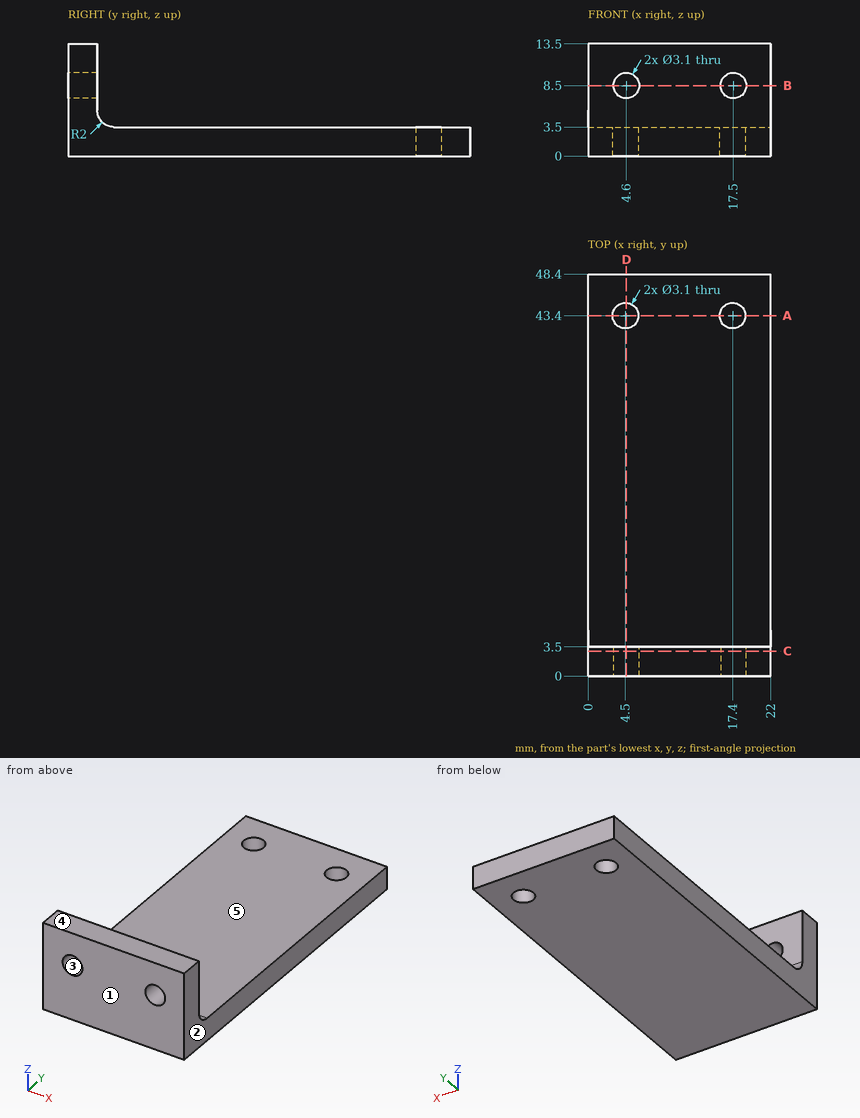
Drawing for the job (mm, zero at the part's lowest x, y, z). A direction names the side the tool comes from. Round coordinates to 2 decimals unless told otherwise and drop trailing zeros. Write each loop counter-clockwise with the first axis right and the second up, starting at its lowest first coordinate (ties: lowest second). Pieces come first, ordered by that corner, then holes. Notation, with made-up numbers: (25, 56) - (31, 56) arc R11 ccw to (31, 64) - close; hole circle Ø8 at (-3.5, 56.25). An arc over 180 degrees is marked (long way). Return JSON: item names as keys, results as strings. Group by question number.
Item 1: Mould opens along X. For the marked faces 1, 2 and 3 say: +X half, -X half, draft (parallel to the pull), parting line (faces both ways), or undercut.
Item 2: Band-saw the part on B-B on z = 8.5. List the corners of the cut face in (x, y), plus the area to 3 significant figures.
Item 3: Band-saw the part on D-D on x = 4.6. List the corners of the cut face in (y, z).
Item 4: Band-saw the part on C-C on y = 3. List the corners of the cut face in (x, z).
Item 5: Band-saw the part on A-A on y = 43.4. List the corners of the cut face in (x, z).
Item 6: Flat gauge pins, fed straight in: pin 1 Ø4 at (x, z) = (12.5, 7.5) entering from +Y; pin 2 Ø5 at (x, y) = (19, 21.5) entering from +Z; pin 3 Ø4 at (x, y) = (7.5, 13) entering from -Z. Where does each tip first touch, or does it go through?
Item 7: Probe probe 1 along X at (y, z) = (1.3, 8.5); probe 2 along Y at (x, z) = (4.5, 2.05); probe 3 along Z at (x, y) = (17.5, 2.4). List the from-to ranges inside material, lowest first.
Item 8: 3-axis set-ups, long thin cutter, end or side, ignore diameter. For the marked faces 4 and 5: which of +Z, -Z, +X, -X, +Y, -Y reach the whole face in a straight line?
Resolved:
{
 "1": {"face 1": "draft", "face 2": "+X half", "face 3": "undercut"},
 "2": {"outline": "(0, 0) - (3.05, 0) - (3.05, 3.5) - (0, 3.5) - close; (6.15, 0) - (15.95, 0) - (15.95, 3.5) - (6.15, 3.5) - close; (19.05, 0) - (22, 0) - (22, 3.5) - (19.05, 3.5) - close", "area": "55.3 mm²"},
 "3": {"outline": "(0, 0) - (41.85, 0) - (41.85, 3.5) - (5.5, 3.5) arc R2 cw to (3.5, 5.5) - (3.5, 6.95) - (0, 6.95) - close; (0, 10.05) - (3.5, 10.05) - (3.5, 13.5) - (0, 13.5) - close; (44.95, 0) - (48.4, 0) - (48.4, 3.5) - (44.95, 3.5) - close"},
 "4": {"outline": "(0, 0) - (22, 0) - (22, 13.5) - (0, 13.5) - close; hole circle Ø3.1 at (4.6, 8.5); hole circle Ø3.1 at (17.5, 8.5)"},
 "5": {"outline": "(0, 0) - (2.95, 0) - (2.95, 3.5) - (0, 3.5) - close; (6.05, 0) - (15.85, 0) - (15.85, 3.5) - (6.05, 3.5) - close; (18.95, 0) - (22, 0) - (22, 3.5) - (18.95, 3.5) - close"},
 "6": {"pin 1": "stops at y = 3.5", "pin 2": "stops at z = 3.5", "pin 3": "stops at z = 0"},
 "7": {"probe 1": "x = 0 to 3.05, 6.15 to 15.95, 19.05 to 22", "probe 2": "y = 0 to 41.85, 44.95 to 48.4", "probe 3": "z = 0 to 6.95, 10.05 to 13.5"},
 "8": {"face 4": "+Z, +X, -X, +Y, -Y", "face 5": "+Z, +X, -X, +Y"}
}
